CAD build for the part. Positions are in the model's coordinates, mm. A direction names the side the tool comes from. Coordinates: 2 decimals unless noted, no trailing zeros. Loops run counter-clockwise (first coordinate to the right, second up) from the corner with the lowest first, then second, coordinate; pieces in that order, holes last. Notation, with made-up numbers: (82, -16) -> (130, -16) arc R21 ccw to (130, 7) -> close; hole circle Ø4 at (5, -39.75). An arc over 180 degrees is marked (long way). Write each question's results on one line, items separated by ' | '.
```python
from build123d import *

# Parameters (mm, degrees)
BOSS_EXTRUDE1_DEPTH = 20
SKETCH2_R           = 40
BOSS_EXTRUDE2_DEPTH = 20
SKETCH3_R           = 12.5
SKETCH3_R_2         = 6.25
CUT_EXTRUDE1_DEPTH  = 41
FILLET1_R           = 10


with BuildPart() as part:
    # Sketch1 → Boss-Extrude1 (new body)
    with BuildSketch(Plane.XY):
        with BuildLine():
            Line((37.75, -43), (-37.75, -43))
            ThreePointArc((-37.75, -43), (-41.462310601, -41.462310601), (-43, -37.75))
            Line((-43, -37.75), (-43, 37.75))
            ThreePointArc((-43, 37.75), (-41.462310601, 41.462310601), (-37.75, 43))
            Line((-37.75, 43), (37.75, 43))
            ThreePointArc((37.75, 43), (41.462310601, 41.462310601), (43, 37.75))
            Line((43, 37.75), (43, -37.75))
            ThreePointArc((43, -37.75), (41.462310601, -41.462310601), (37.75, -43))
        make_face()
    extrude(amount=BOSS_EXTRUDE1_DEPTH)

    # Sketch2 → Boss-Extrude2 (add)
    with BuildSketch(Plane.XY.offset(20)):
        Circle(SKETCH2_R)
    extrude(amount=BOSS_EXTRUDE2_DEPTH)

    # Sketch3 → Cut-Extrude1 (cut, through all)
    with BuildSketch(Plane.XY.offset(40)):
        Circle(SKETCH3_R)
        with Locations((-34, 34)):
            Circle(SKETCH3_R_2)
        with Locations((34, 34)):
            Circle(SKETCH3_R_2)
        with Locations((34, -34)):
            Circle(SKETCH3_R_2)
        with Locations((-34, -34)):
            Circle(SKETCH3_R_2)
    extrude(amount=-CUT_EXTRUDE1_DEPTH, mode=Mode.SUBTRACT)

    # Fillet1
    fillet1_edges = [part.edges().sort_by_distance(p)[0] for p in [
        (-40, 0, 40),
    ]]
    fillet(fillet1_edges, radius=FILLET1_R)


solid = part.part
```
Q1. Cut at A-A on z = 10. Write the cut outline in (x, y), and give its area (3 significant figures).
Results are:
outline: (-43, -37.75) arc R5.25 ccw to (-37.75, -43) -> (37.75, -43) arc R5.25 ccw to (43, -37.75) -> (43, 37.75) arc R5.25 ccw to (37.75, 43) -> (-37.75, 43) arc R5.25 ccw to (-43, 37.75) -> close; hole circle Ø12.5 at (-34, -34); hole circle Ø12.5 at (-34, 34); hole circle Ø25 at (0, 0); hole circle Ø12.5 at (34, -34); hole circle Ø12.5 at (34, 34) | area: 6,390 mm^2
Q2. Drop flat-ended pins along their axis: pin 1 (1.5 mm diameter, centred on x = -26.5, z = 27, fed in from -Y); pin 2 (3 mm diameter, centred on x = -0.5, z = 33, fed in from -Y); pin 3 (12 mm diameter, centred on y = 34, z = 28.5, fed in from +X); pin 4 (7.5 mm diameter, centred on x = 34, y = 34, fed in from +Z). Give the stop position or say it passes through.
Results are:
pin 1: y = -30.61 | pin 2: y = -39.88 | pin 3: x = 28.57 | pin 4: through
Q3. Wall check: L1, parallel to Y at x = 34, z = 9.25; L2, parallel to Y at x = 0, z = 23; L3, parallel to Z at x = -18.5, y = 38. Give the ranges that are in metal, low to high. Write a range as from..to.
Results are:
L1: -43..-40.25, -27.75..27.75, 40.25..43 | L2: -40..-12.5, 12.5..40 | L3: 0..20
Q4. Cut at B-B on y = 0. Write the cut outline in (x, z), and give its area (3 significant figures).
Results are:
outline: (-43, 0) -> (-12.5, 0) -> (-12.5, 40) -> (-30, 40) arc R10 ccw to (-40, 30) -> (-40, 20) -> (-43, 20) -> close; (12.5, 0) -> (43, 0) -> (43, 20) -> (40, 20) -> (40, 30) arc R10 ccw to (30, 40) -> (12.5, 40) -> close | area: 2,280 mm^2
Q5. Pull direction Y, two halves, no side cores. Call faces 1 (the cylindrical face through (29.39, -29.78, 10.14)), 2 (the cylindrical face through (-41.421, -41.503, 9.86)), 3 (the flat face through (-1, 43, 10)), 4 (the flat face through (29, -28, 20)): +Y half, -Y half, draft (parallel to the pull), parting line (faces both ways), or undercut.
Results are:
face 1: undercut | face 2: -Y half | face 3: +Y half | face 4: draft
Q6. Which spindle directions (+Z, -Z, +X, -X, +Y, -Y) get a long thin tool onto all of the face, cutting with end or side? Do faces 5 (the flat face through (13, 0, 40)), 6 (the cylindrical face through (-8.67, -39.05, 24.93)). Say none if no direction does.
Results are:
face 5: +Z, +X, -X, +Y, -Y | face 6: +Z
Q7. Cut at D-D on z = 24. Write the cut outline in (x, y), and give its area (3 significant figures).
Results are:
outline: circle Ø80 at (0, 0); hole circle Ø25 at (0, 0) | area: 4,540 mm^2
